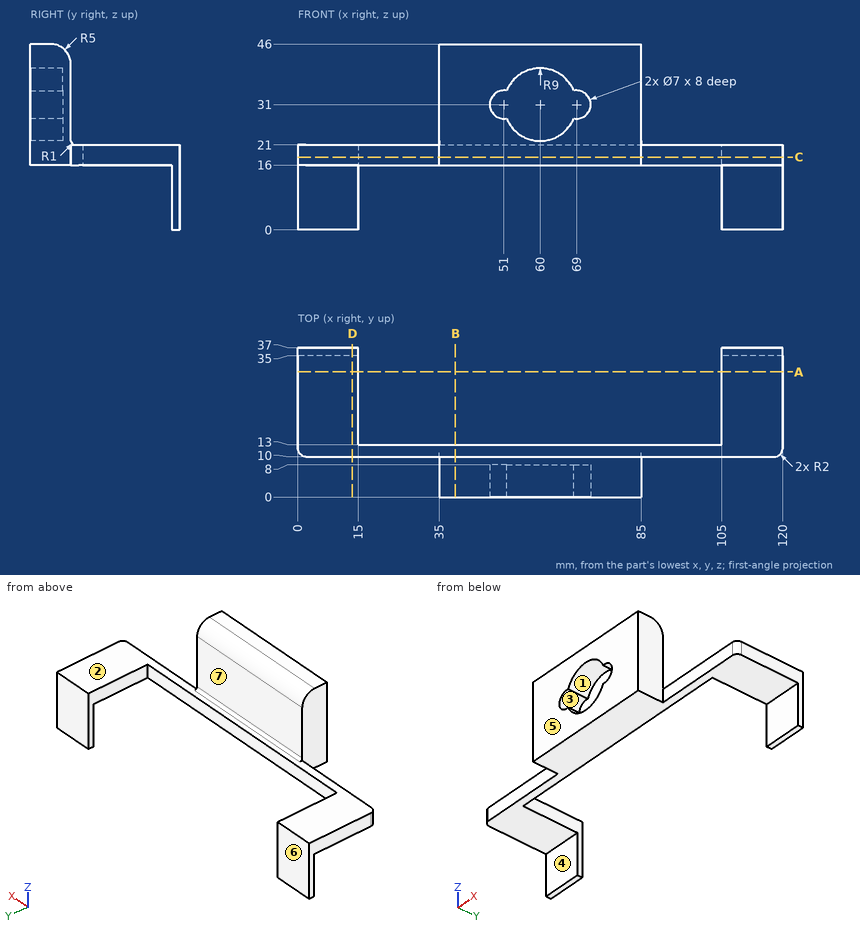
Job drawing, mm, ordinate dimensions from the low corner. One solid piece. A direction names the side the tool comes from. Round coordinates to 2 decimals unless told otherwise and drop trailing zeros. Order: outer loops, then holes, each group sorted by start corner. A loop starts at its lowest first (then second) coordinate and runs counter-clockwise, first axis right, second up. Notation, with made-up numbers: M 8,51.5 L 64,51.5 A18 ccw 64,55.5 Z; hole C 9.5,-3 d3. An arc over 180 degrees is marked long. Write each question's results on one line, items separated by ' | '. Start each with the question number.
(1) Drop flat-ended pins along their axis: pin 1 (6 mm diameter, centred on x = 63.5, y = 6, fed in from -Z); pin 2 (5.5 mm diameter, centred on x = 69, z = 31, fed in from +Y); pin 3 (5.5 mm diameter, centred on y = 5.5, z = 27.5, fed in from -X). Give the stop position or say it passes through.
(2) Saw through at A-A, the plane y = 31. Give the cut face in (x, z).
(3) Two-plate mould, pull along X, no slides. Class the marked faces 1 and 2: pulls with the +X half, pulls with the -X half, needs draft (parallel to the pull), parting line crosses it, or undercut.
(4) Probe probe 1 along X at (y, z) = (4, 31); probe 2 along Z at (x, y) = (69, 3); probe 3 along X at (y, z) = (4.5, 42). List the from-to ranges inside material, lowest first. Write a range as from..to.
(5) Saw through at D-D, the plane x = 13.5. Give the cut face in (y, z).
(6) Saw through at C-C, the plane z = 18. Give the cut face in (x, y).
(7) Saw through at B-B, the plane x = 39. Give the cut face in (y, z).
(8) Which spindle directions (+Z, -Z, +X, -X, +Y, -Y) get a long thin tool onto all of the face, cutting with end or side? Do the marked faces 3, 4, 5, 6 and 7. Say none if no direction does.
Established:
1) pin 1: stops at z = 16 | pin 2: stops at y = 10 | pin 3: stops at x = 35
2) outline: M 0,16 L 15,16 L 15,21 L 0,21 Z; M 105,16 L 120,16 L 120,21 L 105,21 Z
3) face 1: undercut | face 2: needs draft
4) probe 1: x = 35..47.5, 72.5..85 | probe 2: z = 16..27.5, 34.5..46 | probe 3: x = 35..85
5) outline: M 10,16 L 35,16 L 35,0 L 37,0 L 37,21 L 10,21 Z
6) outline: M 0,12 A2 ccw 2,10 L 35,10 L 35,0 L 85,0 L 85,10 L 118,10 A2 ccw 120,12 L 120,37 L 105,37 L 105,13 L 15,13 L 15,37 L 0,37 Z
7) outline: M 0,16 L 13,16 L 13,21 L 11,21 A1 cw 10,22 L 10,41 A5 ccw 5,46 L 0,46 Z
8) face 3: -Y | face 4: -Z, +X, -X, -Y | face 5: +Z, -Z, +X, -X, -Y | face 6: +Z, -Z, +X, -X, +Y | face 7: +Z, +X, -X, +Y
